Geometry: see drawing. Coordinates: mm, zero at the bounding-box minimum. A direction names the side the tool comes from. Give positions to 0.01 mm unless a question says otherwise; leave off trailing zeros. Order: outer loops, then holes, each group sorted by start corner. A loop starts at its lowest first (then second) coordinate and runs counter-clockwise, first axis right, second up. Notation, with made-up numbers: (51.25, 34.5) - (79.25, 34.5) arc R38 cw to (79.25, 72.5) - close; hole circle Ø3 at (-8, 14). An arc over 180 degrees is marked (long way). One line per item, written item: value.
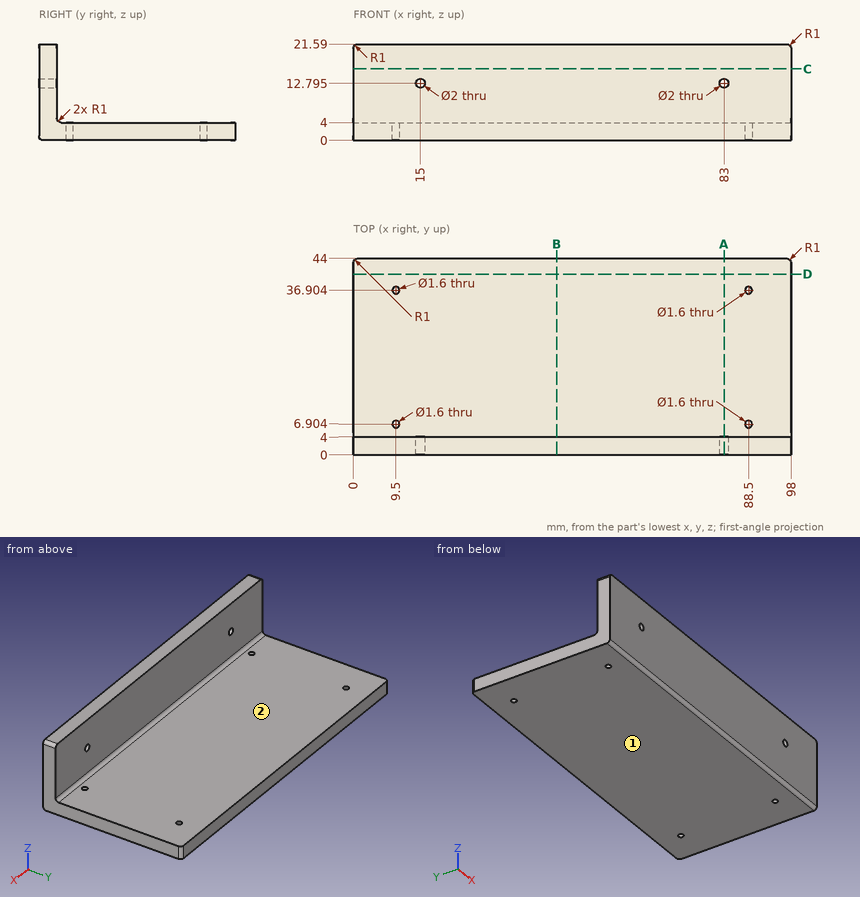
1) Section A-A, the plane x = 83. Return loops of the section in (y, z) (3 decimals).
Answers below:
outline: (0, 1) arc R1 ccw to (1, 0) - (44, 0) - (44, 4) - (5, 4) arc R1 cw to (4, 5) - (4, 11.795) - (0, 11.795) - close; (0, 13.795) - (4, 13.795) - (4, 21.59) - (0, 21.59) - close
2) Section C-C, the plane z = 16. Return loops of the section in (x, y), then the cut area to 3 significant figures.
Answers below:
outline: (0, 0) - (98, 0) - (98, 4) - (0, 4) - close
area: 392 mm^2
3) Set-up query: the marked faces 1 and 2. Return all of +Z, -Z, +X, -X, +Y, -Y with unobstructed straight access to the full face (end or side cutting, diameter ignored); none if empty.
Answers below:
face 1: -Z, +X, -X, +Y, -Y
face 2: +Z, +X, -X, +Y
4) Material intervals for line 1 along Y through (x, z) = (9.5, 0.9) (3 decimals); line 2 along Y through (x, z) = (67, 15), sorted ascending.
Answers below:
line 1: 0.005 to 6.104, 7.704 to 36.104, 37.704 to 44
line 2: 0 to 4
5) First-contact query: pin 1 (10 mm diameter, centred on x = 32, y = 32, fed in from +Z); pin 2 (5 mm diameter, centred on x = 32, z = 16.5, fed in from +Y). Flat tips, straight axial feed; report the tip coordinate or a pass-through.
Answers below:
pin 1: z = 4
pin 2: y = 4
6) Section B-B, the plane x = 45.5. Return loops of the section in (y, z), then the cut area to 3 significant figures.
Answers below:
outline: (0, 1) arc R1 ccw to (1, 0) - (44, 0) - (44, 4) - (5, 4) arc R1 cw to (4, 5) - (4, 21.59) - (0, 21.59) - close
area: 246 mm^2
